from build123d import *

# Parameters (mm, degrees)
BOSS_EXTRUDE1_DEPTH = 20
SKETCH2_W           = 15
SKETCH2_H           = 15
BOSS_EXTRUDE2_DEPTH = 33
SKETCH3_W           = 15
SKETCH3_H           = 15
BOSS_EXTRUDE3_DEPTH = 33
SKETCH4_R           = 2.75
SKETCH4_R_2         = 2.825
CUT_EXTRUDE1_DEPTH  = 73.844011422
CUT_EXTRUDE2_DEPTH  = 74.484692283
SKETCH6_W           = 10
SKETCH6_H           = 10
CUT_EXTRUDE3_DEPTH  = 33
SKETCH7_W           = 10
SKETCH7_H           = 10
CUT_EXTRUDE4_DEPTH  = 33
CHAMFER1_SIZE       = 0.5


with BuildPart() as part:
    # Sketch1 → Boss-Extrude1 (new body)
    with BuildSketch(Plane(origin=(0, 0, 0), x_dir=(1, 0, 0), z_dir=(0, 1, 0))):
        with BuildLine():
            Line((0, 50), (0, 30))
            ThreePointArc((0, 30), (-21.213203436, 21.213203436), (-30, 0))
            Line((-30, 0), (-50, 0))
            ThreePointArc((-50, 0), (-35.355339059, 35.355339059), (0, 50))
        make_face()
    extrude(amount=BOSS_EXTRUDE1_DEPTH)

    # Sketch2 → Boss-Extrude2 (add)
    with BuildSketch(Plane.XY):
        with Locations((-40, 10)):
            Rectangle(SKETCH2_W, SKETCH2_H)
    extrude(amount=BOSS_EXTRUDE2_DEPTH)

    # Sketch3 → Boss-Extrude3 (add)
    with BuildSketch(Plane(origin=(0, 0, 0), x_dir=(0, 0, -1), z_dir=(1, 0, 0))):
        with Locations((40, 10)):
            Rectangle(SKETCH3_W, SKETCH3_H)
    extrude(amount=BOSS_EXTRUDE3_DEPTH)

    # Sketch4 → Cut-Extrude1 (cut, through all)
    with BuildSketch(Plane(origin=(0, 17.5, 0), x_dir=(1, 0, 0), z_dir=(0, 1, 0))):
        with Locations(Location((10, 40, 0), (0, 0, 270))):
            Circle(SKETCH4_R)
        with Locations(Location((25, 40, 0), (0, 0, 270))):
            Circle(SKETCH4_R_2)
        with Locations(Location((-40, -10, 0), (0, 0, 270))):
            Circle(SKETCH4_R)
        with Locations(Location((-40, -25, 0), (0, 0, 270))):
            Circle(SKETCH4_R)
    extrude(amount=-CUT_EXTRUDE1_DEPTH, mode=Mode.SUBTRACT)

    # Sketch5 → Cut-Extrude2 (cut, through all)
    with BuildSketch(Plane(origin=(0, 20, 0), x_dir=(1, 0, 0), z_dir=(0, 1, 0))):
        with BuildLine():
            Line((-21.990223117, 27.155663999), (-28.291433976, 34.937011371))
            ThreePointArc((-28.291433976, 34.937011371), (-29.68093252, 35.671569812), (-31.172202606, 35.17518706))
            ThreePointArc((-31.172202606, 35.17518706), (-33.234018716, 33.234018716), (-35.17518706, 31.172202606))
            ThreePointArc((-35.17518706, 31.172202606), (-35.671569812, 29.68093252), (-34.937011371, 28.291433976))
            Line((-34.937011371, 28.291433976), (-27.155663999, 21.990223117))
            ThreePointArc((-27.155663999, 21.990223117), (-25.744904759, 21.550308438), (-24.417193319, 22.199114181))
            ThreePointArc((-24.417193319, 22.199114181), (-23.334523779, 23.334523779), (-22.199114181, 24.417193319))
            ThreePointArc((-22.199114181, 24.417193319), (-21.550308438, 25.744904759), (-21.990223117, 27.155663999))
        make_face()
        with BuildLine():
            Line((-20.538868638, 28.26932746), (-26.424199651, 36.369790662))
            ThreePointArc((-26.424199651, 36.369790662), (-26.774099933, 37.902060905), (-25.908661914, 39.214043885))
            ThreePointArc((-25.908661914, 39.214043885), (-23.5, 40.703193978), (-21.006027233, 42.044581338))
            ThreePointArc((-21.006027233, 42.044581338), (-19.437097633, 42.138081158), (-18.285062818, 41.068923503))
            Line((-18.285062818, 41.068923503), (-14.21252141, 31.921845736))
            ThreePointArc((-14.21252141, 31.921845736), (-14.152727818, 30.445298653), (-15.123063049, 29.330751167))
            ThreePointArc((-15.123063049, 29.330751167), (-16.5, 28.578838325), (-17.839644098, 27.762332367))
            ThreePointArc((-17.839644098, 27.762332367), (-19.290038151, 27.47927115), (-20.538868638, 28.26932746))
        make_face()
        with BuildLine():
            Line((-12.522383321, 32.621923854), (-16.110622392, 41.969606219))
            ThreePointArc((-16.110622392, 41.969606219), (-16.05201939, 43.540226476), (-14.876504274, 44.583512878))
            ThreePointArc((-14.876504274, 44.583512878), (-12.16449512, 45.398513836), (-9.408325818, 46.04870688))
            ThreePointArc((-9.408325818, 46.04870688), (-7.868656664, 45.73295191), (-7.032594847, 44.402056368))
            Line((-7.032594847, 44.402056368), (-5.466259855, 34.512606439))
            ThreePointArc((-5.466259855, 34.512606439), (-5.790662187, 33.070895758), (-7.016400163, 32.245466794))
            ThreePointArc((-7.016400163, 32.245466794), (-8.541028488, 31.875552268), (-10.046352613, 31.433593482))
            ThreePointArc((-10.046352613, 31.433593482), (-11.52058732, 31.535566946), (-12.522383321, 32.621923854))
        make_face()
        with BuildLine():
            Line((-31.921845736, 14.21252141), (-41.068923503, 18.285062818))
            ThreePointArc((-41.068923503, 18.285062818), (-42.138081158, 19.437097633), (-42.044581338, 21.006027233))
            ThreePointArc((-42.044581338, 21.006027233), (-40.703193978, 23.5), (-39.214043885, 25.908661914))
            ThreePointArc((-39.214043885, 25.908661914), (-37.902060905, 26.774099933), (-36.369790662, 26.424199651))
            Line((-36.369790662, 26.424199651), (-28.26932746, 20.538868638))
            ThreePointArc((-28.26932746, 20.538868638), (-27.47927115, 19.290038151), (-27.762332367, 17.839644098))
            ThreePointArc((-27.762332367, 17.839644098), (-28.578838325, 16.5), (-29.330751167, 15.123063049))
            ThreePointArc((-29.330751167, 15.123063049), (-30.445298653, 14.152727818), (-31.921845736, 14.21252141))
        make_face()
        with BuildLine():
            Line((-34.512606439, 5.466259855), (-44.402056368, 7.032594847))
            ThreePointArc((-44.402056368, 7.032594847), (-45.73295191, 7.868656664), (-46.04870688, 9.408325818))
            ThreePointArc((-46.04870688, 9.408325818), (-45.398513836, 12.16449512), (-44.583512878, 14.876504274))
            ThreePointArc((-44.583512878, 14.876504274), (-43.540226476, 16.05201939), (-41.969606219, 16.110622392))
            Line((-41.969606219, 16.110622392), (-32.621923854, 12.522383321))
            ThreePointArc((-32.621923854, 12.522383321), (-31.535566946, 11.52058732), (-31.433593482, 10.046352613))
            ThreePointArc((-31.433593482, 10.046352613), (-31.875552268, 8.541028488), (-32.245466794, 7.016400163))
            ThreePointArc((-32.245466794, 7.016400163), (-33.070895758, 5.790662187), (-34.512606439, 5.466259855))
        make_face()
    extrude(amount=-CUT_EXTRUDE2_DEPTH, mode=Mode.SUBTRACT)

    # Sketch6 → Cut-Extrude3 (cut)
    with BuildSketch(Plane(origin=(33, 0, 0), x_dir=(0, 0, -1), z_dir=(1, 0, 0))):
        with Locations((40, 10)):
            Rectangle(SKETCH6_W, SKETCH6_H)
    extrude(amount=-CUT_EXTRUDE3_DEPTH, mode=Mode.SUBTRACT)

    # Sketch7 → Cut-Extrude4 (cut)
    with BuildSketch(Plane.XY.offset(33)):
        with Locations((-40, 10)):
            Rectangle(SKETCH7_W, SKETCH7_H)
    extrude(amount=-CUT_EXTRUDE4_DEPTH, mode=Mode.SUBTRACT)

    # Chamfer1
    chamfer1_edges = [part.edges().sort_by_distance(p)[0] for p in [
        (-32.5, 10, 33),
        (-40, 17.5, 33),
        (-47.5, 10, 33),
        (-40, 2.5, 33),
        (33, 10, -45),
        (33, 15, -40),
        (33, 10, -35),
        (33, 5, -40),
        (-35, 10, 33),
        (-40, 15, 33),
        (-45, 10, 33),
        (-40, 5, 33),
        (33, 10, -47.5),
        (33, 17.5, -40),
        (33, 10, -32.5),
        (33, 2.5, -40),
    ]]
    chamfer(chamfer1_edges, length=CHAMFER1_SIZE)


solid = part.part
Read the model definition and answer for the solid it produces. Units are mm, in the model's axes. A direction names the side the tool comes from. Round coordinates to 2 decimals unless told otherwise and drop trailing zeros. Write each loop counter-clockwise with the first axis right and the second up, starting at its lowest first coordinate (ties: lowest second). Pieces come first, ordered by that corner, then holes. Notation, with made-up numbers: (53, 77.5) - (78, 77.5) arc R36 ccw to (78, 115.5) - close; hole circle Ø5 at (-27.5, 63.25). An arc over 180 degrees is marked (long way). Use a Markdown table: item, result.
(1) Straight lines are drawn through the part: line 1 along X through (y, z) = (4.2, 25); line 2 along X through (y, z) = (9.75, -39); line 3 along X through (y, z) = (16.95, -40) (3 decimals). For each, find the intervals that lie inside material, in ascending order. Write a range as [from, to].
Reported:
| item | result |
|---|---|
| line 1 | [-47.5, -42.75], [-37.25, -32.5] |
| line 2 | [-31.29, -26.18], [-17.36, -14.97], [-6.18, 0] |
| line 3 | [-30, -24.678], [-17.809, -15.355], [-6.335, 7.25], [12.75, 22.175], [27.825, 33] |
(2) Each of these flat-tipped pins is pushed along its axis until it touches: pin 1 Ø4.5 at (x, y) = (18, 7.5) entering from +Z; pin 2 Ø5 at (x, y) = (10.5, 11) entering from -Z; pin 3 Ø4.5 at (x, z) = (-43.5, 13) entering from -Y; pin 4 Ø4.5 at (x, z) = (10, -40) entering from +Y. Where does it stop, or does it pass through?
Reported:
| item | result |
|---|---|
| pin 1 | z = -32.5 |
| pin 2 | z = -47.5 |
| pin 3 | y = 2.5 |
| pin 4 | through |
(3) The part is cut by section A-A (z = 25). Write down the section's boundary in (x, y).
Reported:
| item | result |
|---|---|
| outline | (-47.5, 2.5) - (-42.75, 2.5) - (-42.75, 5) - (-45, 5) - (-45, 15) - (-42.75, 15) - (-42.75, 17.5) - (-47.5, 17.5) - close; (-37.25, 2.5) - (-32.5, 2.5) - (-32.5, 17.5) - (-37.25, 17.5) - (-37.25, 15) - (-35, 15) - (-35, 5) - (-37.25, 5) - close |
(4) The part is cut by section B-B (x = 25). Write down the section's boundary in (y, z) (3 decimals), then the cut area to 4 significant figures.
Reported:
| item | result |
|---|---|
| outline | (2.5, -47.5) - (17.5, -47.5) - (17.5, -42.825) - (15, -42.825) - (15, -45) - (5, -45) - (5, -42.825) - (2.5, -42.825) - close; (2.5, -37.175) - (5, -37.175) - (5, -35) - (15, -35) - (15, -37.175) - (17.5, -37.175) - (17.5, -32.5) - (2.5, -32.5) - close |
| area | 96.75 mm2 |
(5) The part is cut by section C-C (y = 14). State how many separate pieces and enclosed holes the cut face has, then the cut area to 3 significant figures.
Reported:
| item | result |
|---|---|
| separate pieces | 1 |
| enclosed holes | 5 |
| area | 1,020 mm2 |
(6) Which of the six approach directions +Z, -Z, +X, -X, +Y, -Y give full straight-line access (tool end or side, diameter ignored) to faces 4 (the flat face through (33, 10, -46)), 5 (the flat face through (-35, 10, 16)), 6 (the cylindrical face through (-27.483, 10.14, -19.311))?
Reported:
| item | result |
|---|---|
| face 4 | +Z, -Z, +X, +Y, -Y |
| face 5 | +Z |
| face 6 | +Y, -Y |
(7) The mould has two halves that part along X. Classify faces 1 (the flat face through (-23, 0, -29)), 2 (the cylindrical face through (-16.48, 10.14, -28.59)), 3 (the cylindrical face through (-35.742, 9.86, -34.964)): released by +X, released by -X, zero draft, split by the parting line, or undercut.
Reported:
| item | result |
|---|---|
| face 1 | zero draft |
| face 2 | undercut |
| face 3 | released by -X |
